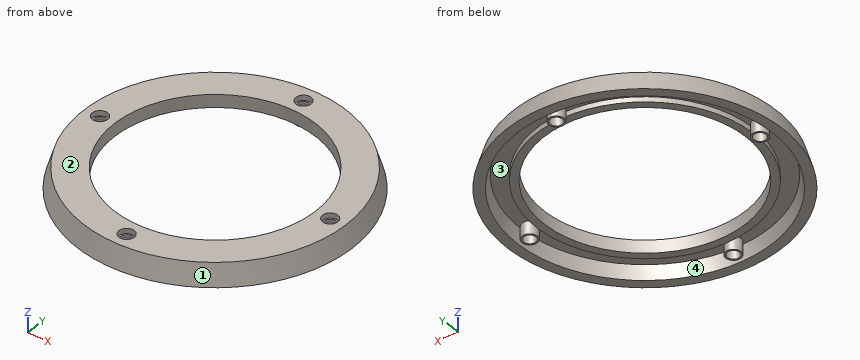
```python
from build123d import *

# Parameters (mm, degrees)
SKETCH001_R              = 1.5
POCKET_DEPTH             = 1
POLARPATTERN_COUNT       = 4
SKETCH002_R              = 1.19
POCKET001_DEPTH          = 155.098074
POLARPATTERN001_COUNT    = 4
SKETCH003_R              = 1.5
PAD_DEPTH                = 2.5
POLARPATTERN002_COUNT    = 4
POLARPATTERN002_FACE38_R = 1.19
POCKET002_DEPTH          = 154.598074
POLARPATTERN003_COUNT    = 4


with BuildPart() as part:
    # Sketch → Revolution (revolve)
    with BuildSketch(Plane.XZ):
        Polygon((19.65, 1.5), (19.65, 4), (25.65, 4), (26.85, 0), (24.9, 0), (24.15, 2.5), (21.15, 2.5), (21.15, 1.5), align=None)
    revolve(axis=Axis((0, 0, 0), (0, 0, 1)))

    # Sketch001 (on Face2 of Revolution) → Pocket (cut)
    with BuildSketch(Plane(origin=(0, 0, 4), x_dir=(-1, 0, 0), z_dir=(0, 0, 1))):
        with Locations((0, 22.65)):
            Circle(SKETCH001_R)
    pocket = extrude(amount=-POCKET_DEPTH, mode=Mode.SUBTRACT)

    # PolarPattern: Pocket ×4 about axis
    polarpattern_axis = Axis((0, 0, 4), (0, 0, 1))
    for i in range(1, POLARPATTERN_COUNT):
        add(pocket.rotate(polarpattern_axis, i * 360 / POLARPATTERN_COUNT), mode=Mode.SUBTRACT)

    # Sketch002 (on Face14 of PolarPattern) → Pocket001 (cut, through all)
    with BuildSketch(Plane(origin=(0, 0, 3), x_dir=(-1, 0, 0), z_dir=(0, 0, 1))):
        with Locations((0, 22.65)):
            Circle(SKETCH002_R)
    pocket001 = extrude(amount=-POCKET001_DEPTH, mode=Mode.SUBTRACT)

    # PolarPattern001: Pocket001 ×4 about axis
    polarpattern001_axis = Axis((0, 0, 3), (0, 0, 1))
    for i in range(1, POLARPATTERN001_COUNT):
        add(pocket001.rotate(polarpattern001_axis, i * 360 / POLARPATTERN001_COUNT), mode=Mode.SUBTRACT)

    # Sketch003 (on Face10 of PolarPattern001) → Pad (join)
    with BuildSketch(Plane(origin=(0, 0, 2.5), x_dir=(1, 0, 0), z_dir=(0, 0, -1))):
        with Locations((0, 22.65)):
            Circle(SKETCH003_R)
    pad = extrude(amount=PAD_DEPTH)

    # PolarPattern002: Pad ×4 about axis
    polarpattern002_axis = Axis((0, 0, 2.5), (0, 0, -1))
    for i in range(1, POLARPATTERN002_COUNT):
        add(pad.rotate(polarpattern002_axis, i * 360 / POLARPATTERN002_COUNT))

    # PolarPattern002 Face38 → Pocket002 (cut, through all)
    with BuildSketch(Plane(origin=(22.65, 0, 2.5), x_dir=(0, 1, 0), z_dir=(0, 0, 1))):
        Circle(POLARPATTERN002_FACE38_R)
    pocket002 = extrude(amount=-POCKET002_DEPTH, mode=Mode.SUBTRACT)

    # PolarPattern003: Pocket002 ×4 about axis
    polarpattern003_axis = Axis((0, 0, 0), (0, 0, 1))
    for i in range(1, POLARPATTERN003_COUNT):
        add(pocket002.rotate(polarpattern003_axis, i * 360 / POLARPATTERN003_COUNT), mode=Mode.SUBTRACT)


solid = part.part
```
Geometry check sheet. Reference: the model listing, model coordinates, mm. Face numbers are marked on the shaded views. Give positions to 0.01 mm unless a question says otherwise; leave off trailing zeros. Use a Markdown table: item, result.
Q1. Draft check along Y on the marked faces 1, 2, 3 and 4. Enter one of: pulls with the +Y half, pulls with the -Y half, needs draft (parallel to the pull), parting line crosses it, or undercut.
Computed:
| item | result |
|---|---|
| face 1 | parting line crosses it |
| face 2 | needs draft |
| face 3 | undercut |
| face 4 | undercut |
Q2. Thickness scan on L1, parallel to Y at x = 10.5, z = 1.95; L2, parallel to Y at x = 0, z = 3.55 (3 decimals); L3, parallel to X at y = -17, z = 2.15. Record the ranges inside material, lowest first. Write a range as [from, to].
Computed:
| item | result |
|---|---|
| L1 | y = [-24.07, -21.93], [-18.36, -16.61], [16.61, 18.36], [21.93, 24.07] |
| L2 | y = [-25.785, -24.15], [-21.15, -19.65], [19.65, 21.15], [24.15, 25.785] |
| L3 | x = [-19.94, -17.3], [-12.58, -9.86], [9.86, 12.58], [17.3, 19.94] |
Q3. Go/stop test with flat-tipped pins: P1, Ø12, axis at x = 9, y = -12, coming from the -Z side; P2, Ø4, axis at x = -22.65, y = 0, coming from the -Z side; P3, Ø1.9, axis at x = 22.65, y = 0, coming from the -Z side; P4, Ø2, axis at y = 1, z = 0.5, coming from the +X side. Record where each tip stops, or that it passes through.
Computed:
| item | result |
|---|---|
| P1 | stops at z = 1.5 |
| P2 | stops at z = 0 |
| P3 | passes through |
| P4 | stops at x = 26.85 |
